```python
from build123d import *

# Parameters (mm, degrees)
F15_R     = 2.5
F0_DEPTH  = 4.5
F3_W      = 2.5
F3_H      = 7
F4_DEPTH  = 3.5
F5_R      = 4
F6_DEPTH  = 2
F7_R      = 2
F8_DEPTH  = 13
F11_W     = 1
F11_H     = 11
F12_DEPTH = 12.5
F13_W     = 11
F13_H     = 5
F14_DEPTH = 25


with BuildPart() as f0:
    # F15 (on Front) → F0 (new body)
    with BuildSketch(Plane.XZ):
        Circle(F15_R)
    extrude(amount=F0_DEPTH)

    # F1 (on Right) → F2 (revolve)
    with BuildSketch(Plane.YZ):
        Polygon((-6.5, 0), (-4.5, 0), (-4.5, 2.5), (-5.202062, 3.0891), (-6.5, 2), align=None)
    revolve(axis=Axis((0, -8.987078, 0), (0, -1, 0)))

    # F3 (on Top) → F4 (cut, symmetric)
    with BuildSketch(Plane.XY):
        with Locations((0, -5.5)):
            Rectangle(F3_W, F3_H)
    extrude(amount=F4_DEPTH, both=True, mode=Mode.SUBTRACT)

    # F5 (on face) → F6 (join)
    with BuildSketch(Plane.XZ):
        Circle(F5_R)
    extrude(amount=-F6_DEPTH)

    # F7 (on face) → F8 (join)
    with BuildSketch(Plane(origin=(0, 2, 0), x_dir=(-1, 0, 0), z_dir=(0, 1, 0))):
        Circle(F7_R)
    extrude(amount=F8_DEPTH)

    # F9 (on Right) → F10 (revolve)
    with BuildSketch(Plane.YZ):
        Polygon((15, 2), (15, 0), (17, 0), (17, 1.5), (15.196913, 2.541013), align=None)
    revolve(axis=Axis((0, 16, 0), (0, 1, 0)))

    # F11 (on Top) → F12 (cut, symmetric)
    with BuildSketch(Plane.XY):
        with Locations((0, 12.5)):
            Rectangle(F11_W, F11_H)
    extrude(amount=F12_DEPTH, both=True, mode=Mode.SUBTRACT)

    # F13 (on Front) → F14 (cut, symmetric)
    with BuildSketch(Plane.XZ):
        with Locations((0, 4)):
            Rectangle(F13_W, F13_H)
        with Locations((0, -4)):
            Rectangle(F13_W, F13_H)
    extrude(amount=F14_DEPTH, both=True, mode=Mode.SUBTRACT)


solid = f0.part
```
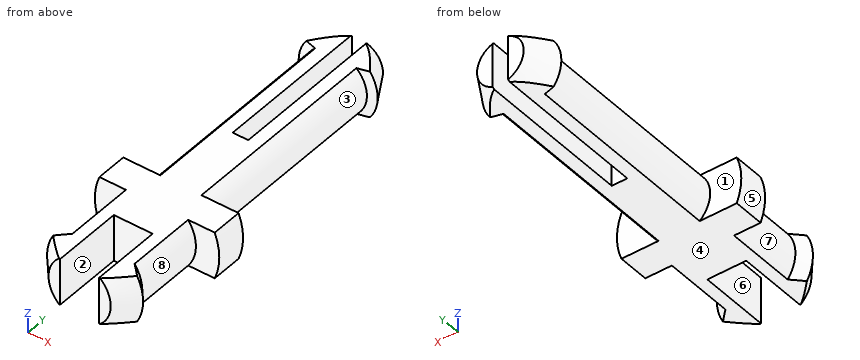
Work out the finished part from the listing and answer in its coordinate system (mm). Face numbers are marked on the shaded views. A direction names the side the tool comes from. Give positions to 0.01 mm unless a question says otherwise; leave off trailing zeros. Loops run counter-clockwise (first coordinate to the right, second up) from the corner with the lowest first, then second, coordinate; pieces in that order, holes last. Notation, with made-up numbers: (51, 44) -> (56, 44) arc R16 ccw to (56, 70) -> close; hole circle Ø6 at (22.25, 75). An arc over 180 degrees is marked (long way). Write item = value, one per line. Start each with the question number.
(1) Which of the six approach directions +Z, -Z, +X, -X, +Y, -Y give full straight-line access (tool end or side, diameter ignored) to the marked faces 4, 5, 6, 7 and 8?
(2) Find section D-D on y = -1. Give the vertices of the cut face in (x, z), and give its area (3 significant figures).
(3) Find section A-A on y = 7.5. Give the vertices of the cut face in (x, z), and give its area (3 significant figures).
(4) Given pin 1 Ø0.5 at (x, z) = (0, -0.5) entering from +Y; pin 2 Ø1.6 at (x, z) = (3, 0) entering from -Y; pin 3 Ø0.9 at (y, z) = (9.5, 0.5) entering from +X, each flat-ended and moving along its own axis, determine where each tip first touches the part or whether it passes through.
(5) Find the intervals of material crossed by probe 1 along X at (y, z) = (8.5, -0.8); probe 2 along X at (y, z) = (8.5, -0.15); probe 3 along Y at (x, z) = (3.75, -0.2), in increasing order. Write a range as from..to.
(6) Find section B-B on z = 0. Give the vertices of the cut face in (x, y), and give its area (3 significant figures).
(7) The mould has two halves that part along X. Classify the marked faces 1, 2 and 3: +X half, -X half, draft (parallel to the pull), parting line (faces both ways), or undercut.
(8) Find section C-C on y = -3.5. Give the vertices of the cut face in (x, z), and give its area (3 significant figures).
From the geometry:
q1.face_4 = -Z, +X, -X, +Y, -Y
q1.face_5 = -X, +Y, -Y
q1.face_6 = +Z, -Z, -Y
q1.face_7 = -X
q1.face_8 = +X
q2.outline = (-2, -1.5) -> (2, -1.5) arc R2.5 ccw to (2, 1.5) -> (-2, 1.5) arc R2.5 ccw to start
q2.area = 14.0 mm^2
q3.outline = (-1.32, -1.5) -> (-0.5, -1.5) -> (-0.5, 1.5) -> (-1.32, 1.5) arc R2 ccw to start; (0.5, -1.5) -> (1.32, -1.5) arc R2 ccw to (1.32, 1.5) -> (0.5, 1.5) -> close
q3.area = 7.75 mm^2
q4.pin_1 = 7
q4.pin_2 = -6.26
q4.pin_3 = 2
q5.probe_1 = -1.83..-0.5, 0.5..1.83
q5.probe_2 = -1.99..-0.5, 0.5..1.99
q5.probe_3 = 0..2
q6.outline = (-4, 0) -> (-2.5, 0) -> (-2.5, -4.5) -> (-3.09, -5.2) -> (-2, -6.5) -> (-1.25, -6.5) -> (-1.25, -2) -> (1.25, -2) -> (1.25, -6.5) -> (2, -6.5) -> (3.09, -5.2) -> (2.5, -4.5) -> (2.5, 0) -> (4, 0) -> (4, 2) -> (2, 2) -> (2, 15) -> (2.54, 15.2) -> (1.5, 17) -> (0.5, 17) -> (0.5, 7) -> (-0.5, 7) -> (-0.5, 17) -> (-1.5, 17) -> (-2.54, 15.2) -> (-2, 15) -> (-2, 2) -> (-4, 2) -> close
q6.area = 88.0 mm^2
q7.face_1 = draft
q7.face_2 = undercut
q7.face_3 = +X half
q8.outline = (-2, -1.5) -> (-1.25, -1.5) -> (-1.25, 1.5) -> (-2, 1.5) arc R2.5 ccw to start; (1.25, -1.5) -> (2, -1.5) arc R2.5 ccw to (2, 1.5) -> (1.25, 1.5) -> close
q8.area = 6.54 mm^2
